from build123d import *

# Parameters (mm, degrees)
F0_R     = 57.329977
F0_R_2   = 53.180957
F1_DEPTH = 32.512
F2_R     = 53.391542
F2_R_2   = 51.816
F3_DEPTH = 13.081
F4_SIZE  = 0.762


with BuildPart() as f1:
    # F0 (on Front) → F1 (new body)
    with BuildSketch(Plane.XZ):
        Circle(F0_R)
        Circle(F0_R_2, mode=Mode.SUBTRACT)
    extrude(amount=F1_DEPTH)

    # F2 (on Front) → F3 (join)
    with BuildSketch(Plane.XZ):
        Circle(F2_R)
        Circle(F2_R_2, mode=Mode.SUBTRACT)
    extrude(amount=F3_DEPTH)

    # F4
    f4_edges = [f1.edges().sort_by_distance(p)[0] for p in [
        (-53.180957, -32.512, 0),
        (-51.816, 0, 0),
        (-57.329977, -32.512, 0),
        (-57.329977, 0, 0),
    ]]
    chamfer(f4_edges, length=F4_SIZE)


solid = f1.part
Geometry: final body of the model. Coordinates: model frame, mm. A direction names the side the tool comes from. Give positions to 0.01 mm unless a question says otherwise; leave off trailing zeros. Write each loop counter-clockwise with the first axis right and the second up, starting at its lowest first coordinate (ties: lowest second). Pieces come first, ordered by that corner, then holes. Notation, with made-up numbers: (33.25, 48.5) -> (66.25, 48.5) arc R27 ccw to (66.25, 65.5) -> close; hole circle Ø9 at (38, 31). An arc over 180 degrees is marked (long way). Answer in a Markdown table with one row per item.
(1) Pin query (flat end, axial travel): pin 1 (3 mm diameter, centred on y = -28.5, z = -29, fed in from +X); pin 2 (2 mm diameter, centred on x = -21.5, y = -17.5, fed in from +Z); pin 3 (2 mm diameter, centred on y = -6, z = -11, fed in from +X). Return the tip coordinate at first contact, or that it passes through.
Answers below:
| item | result |
|---|---|
| pin 1 | x = 50.3 |
| pin 2 | z = 53.54 |
| pin 3 | x = 56.45 |
(2) Ray query, line 1 along Z through (x, y) = (0, -16.75); line 2 along Z through (x, y) = (0, -5.75); line 3 along X through (y, z) = (-5, 33). Return the intervals inside material, ascending. Write a range as [from, to].
Answers below:
| item | result |
|---|---|
| line 1 | [-57.33, -53.18], [53.18, 57.33] |
| line 2 | [-57.33, -51.82], [51.82, 57.33] |
| line 3 | [-46.88, -39.95], [39.95, 46.88] |
(3) Section query B-B on x = 0. Return loops of the section in (y, z).
Answers below:
| item | result |
|---|---|
| outline | (-32.51, -56.57) -> (-31.75, -57.33) -> (-0.76, -57.33) -> (0, -56.57) -> (0, -52.58) -> (-0.76, -51.82) -> (-13.08, -51.82) -> (-13.08, -53.18) -> (-31.75, -53.18) -> (-32.51, -53.94) -> close; (-32.51, 53.94) -> (-31.75, 53.18) -> (-13.08, 53.18) -> (-13.08, 51.82) -> (-0.76, 51.82) -> (0, 52.58) -> (0, 56.57) -> (-0.76, 57.33) -> (-31.75, 57.33) -> (-32.51, 56.57) -> close |
(4) Section query A-A on z = 0. Return loops of the section in (x, y), then the cut area to 3 significant figures.
Answers below:
| item | result |
|---|---|
| outline | (-57.33, -31.75) -> (-56.57, -32.51) -> (-53.94, -32.51) -> (-53.18, -31.75) -> (-53.18, -13.08) -> (-51.82, -13.08) -> (-51.82, -0.76) -> (-52.58, 0) -> (-56.57, 0) -> (-57.33, -0.76) -> close; (51.82, -13.08) -> (53.18, -13.08) -> (53.18, -31.75) -> (53.94, -32.51) -> (56.57, -32.51) -> (57.33, -31.75) -> (57.33, -0.76) -> (56.57, 0) -> (52.58, 0) -> (51.82, -0.76) -> close |
| area | 303 mm^2 |
(5) Section query C-C on y = -30. Return loops of the section in (x, z).
Answers below:
| item | result |
|---|---|
| outline | circle Ø114.66 at (0, 0); hole circle Ø106.36 at (0, 0) |
(6) Set-up query: faces 1 (the cylindrical face through (50.725, -22.285, 15.974)), 2 (the cylindrical face through (-11.233, -6.835, -50.584)). Return all of +Z, -Z, +X, -X, +Y, -Y with unobstructed straight access to the full face (end or side cutting, diameter ignored); none if empty.
Answers below:
| item | result |
|---|---|
| face 1 | -Y |
| face 2 | +Y, -Y |
